The listing builds one solid part. Answer for the finished solid, in the listing's coordinates (mm). Face numbers are marked on the shaded views. A direction names the side the tool comes from. Round coordinates to 2 decimals unless told otherwise and drop trailing zeros. Order: outer loops, then holes, each group sorted by start corner. A loop starts at its lowest first (then second) coordinate and runs counter-clockwise, first axis right, second up. Notation, with made-up numbers: (-16.5, 84) -> (1.5, 84) arc R9 ccw to (1.5, 90) -> close; hole circle Ø8 at (-1.75, 81.25). An arc over 180 degrees is marked (long way). Answer in a Markdown table with one row per item. Add a question column.
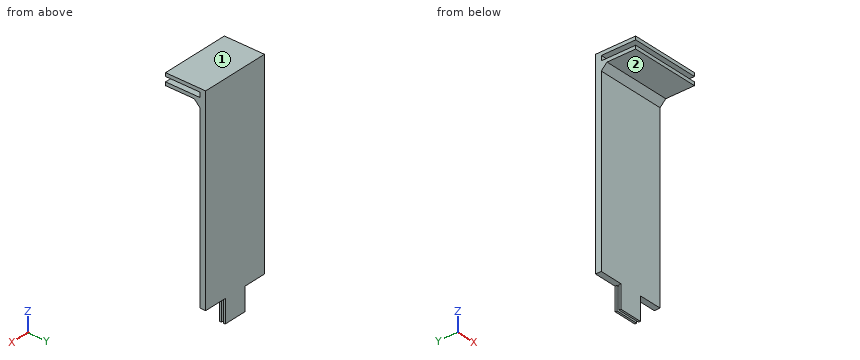
```python
from build123d import *

# Parameters (mm, degrees)
SKETCH1_W                = 20
SKETCH1_H                = 80
BOSS_EXTRUDE1_DEPTH      = 5
BOSS_EXTRUDE2_DEPTH      = 30
BOSS_EXTRUDE2_DEPTH_BACK = 5
SKETCH2_W                = 20
SKETCH2_H                = 10.2
SKETCH3_W                = 20
SKETCH3_H                = 4.2
CUT_EXTRUDE1_DEPTH       = 30
BOSS_EXTRUDE3_DEPTH      = 40
SKETCH6_W                = 60
SKETCH6_H                = 5
BOSS_EXTRUDE4_DEPTH      = 81.9
SKETCH7_W                = 20
SKETCH7_H                = 1.65
BOSS_EXTRUDE5_DEPTH      = 20
CHAMFER1_SIZE            = 5


with BuildPart() as part:
    # Sketch1 → Boss-Extrude1 (new body)
    with BuildSketch(Plane(origin=(0, 0, 0), x_dir=(1, 0, 0), z_dir=(0, 1, 0))):
        with Locations((10, 40)):
            Rectangle(SKETCH1_W, SKETCH1_H)
    extrude(amount=BOSS_EXTRUDE1_DEPTH)

    # Sketch2 → Boss-Extrude2 (add, two sides: drawn at the far end of the back side and taken through both)
    with BuildSketch(Plane.XZ.offset(-BOSS_EXTRUDE2_DEPTH_BACK)):
        with Locations((10, 5.1)):
            Rectangle(SKETCH2_W, SKETCH2_H)
    extrude(amount=BOSS_EXTRUDE2_DEPTH + BOSS_EXTRUDE2_DEPTH_BACK)

    # Sketch3 → Cut-Extrude1 (cut)
    with BuildSketch(Plane.XZ.offset(30)):
        with Locations((10, 5.1)):
            Rectangle(SKETCH3_W, SKETCH3_H)
    extrude(amount=-CUT_EXTRUDE1_DEPTH, mode=Mode.SUBTRACT)

    # Sketch5 → Boss-Extrude3 (add)
    with BuildSketch(Plane.ZY):
        Polygon((3, 0), (7.2, 0), (7.2, 5), (-80, 5), (-80, 0), (0, 0), (0, -30), (3, -30), align=None)
        Polygon((7.2, -30), (10.2, -30), (10.2, 5), (7.2, 5), (7.2, 0), align=None)
    extrude(amount=BOSS_EXTRUDE3_DEPTH)

    # Sketch6 → Boss-Extrude4 (add)
    with BuildSketch(Plane(origin=(0, 0, -80), x_dir=(-1, 0, 0), z_dir=(0, 0, -1))):
        with Locations((10, 2.5)):
            Rectangle(SKETCH6_W, SKETCH6_H)
    extrude(amount=BOSS_EXTRUDE4_DEPTH)

    # Sketch7 → Boss-Extrude5 (add)
    with BuildSketch(Plane(origin=(0, 0, -161.9), x_dir=(-1, 0, 0), z_dir=(0, 0, -1))):
        with Locations((10, 4.175)):
            Rectangle(SKETCH7_W, SKETCH7_H)
        with Locations((10, 0.825)):
            Rectangle(SKETCH7_W, SKETCH7_H)
    extrude(amount=BOSS_EXTRUDE5_DEPTH)

    # Chamfer1
    chamfer1_edges = [part.edges().sort_by_distance(p)[0] for p in [
        (-10, 0, 0),
    ]]
    chamfer(chamfer1_edges, length=CHAMFER1_SIZE)


solid = part.part
```
Item 1: Flat-ended cylindrical pins translate along their axes: P1, Ø10, axis at x = -8.5, z = -171.5, coming from the -Y side; P2, Ø12.5, axis at x = -11.5, y = -19, coming from the -Z side; P3, Ø1.3, axis at y = 1, z = -168, coming from the +X side. Find the tip coordinate at first contact, or state that the pin passes through.
Item 2: The part is cut by section C-C, the plane y = -12.5. Give the vertices of the cut face in (x, z), and give its area (3 significant figures).
Item 3: The part is cut by section A-A, the plane y = -2. Give the vertices of the cut face in (x, z).
Item 4: The part is cut by section B-B, the plane x = 9. Give the vertices of the cut face in (y, z), and give its area (3 significant figures).
Item 5: A tool of negligible diameter and unlimited length cuts with its end or side. For the marked faces 1 and 2, from which of +Z, -Z, +X, -X, +Y, -Y can it reach the whole face along a straight path? Write none if from no direction.
Item 6: Find the intervals of material crossed by probe 1 along Z at (x, y) = (14.5, -6.5); probe 2 along Z at (x, y) = (5, 1.5); probe 3 along Y at (x, z) = (10, -7), in increasing order. Write a range as [from, to].
Item 7: The part is cut by section D-D, the plane z = -114. Give the vertices of the cut face in (x, y), and give its area (3 significant figures).
Resolved:
| question | item | result |
|---|---|---|
| 1 | P1 | y = 0 |
| 1 | P2 | z = 0 |
| 1 | P3 | x = 0 |
| 2 | outline | (-40, 0) -> (20, 0) -> (20, 3) -> (-40, 3) -> close; (-40, 7.2) -> (20, 7.2) -> (20, 10.2) -> (-40, 10.2) -> close |
| 2 | area | 360 mm2 |
| 3 | outline | (-40, -3) -> (20, -3) -> (20, 3) -> (-40, 3) -> close; (-40, 7.2) -> (20, 7.2) -> (20, 10.2) -> (-40, 10.2) -> close |
| 4 | outline | (-30, 0) -> (-5, 0) -> (0, -5) -> (0, -161.9) -> (5, -161.9) -> (5, 10.2) -> (-30, 10.2) -> (-30, 7.2) -> (0, 7.2) -> (0, 3) -> (-30, 3) -> close |
| 4 | area | 1,050 mm2 |
| 5 | face 1 | +Z, +X, -X, +Y, -Y |
| 5 | face 2 | -Z, +X, -X, -Y |
| 6 | probe 1 | [0, 3], [7.2, 10.2] |
| 6 | probe 2 | [-161.9, 10.2] |
| 6 | probe 3 | [0, 5] |
| 7 | outline | (-40, 0) -> (20, 0) -> (20, 5) -> (-40, 5) -> close |
| 7 | area | 300 mm2 |
